Verification items for this drawing (mm, ordinates from the low corner). A direction names the side the tool comes from. Give positions to 0.01 mm unless a question says otherwise; leave off trailing zeros. Order: outer loops, then holes, each group sorted by start corner. A loop starts at its lowest first (then second) coordinate and runs counter-clockwise, first axis right, second up. Notation, with made-up numbers: M 36,68.5 L 71,68.5 A28 ccw 71,98.5 Z; hole C 84.5,-37.5 d9. An arc over 180 degrees is marked long. Answer as a JSON object with one key per item and string values.
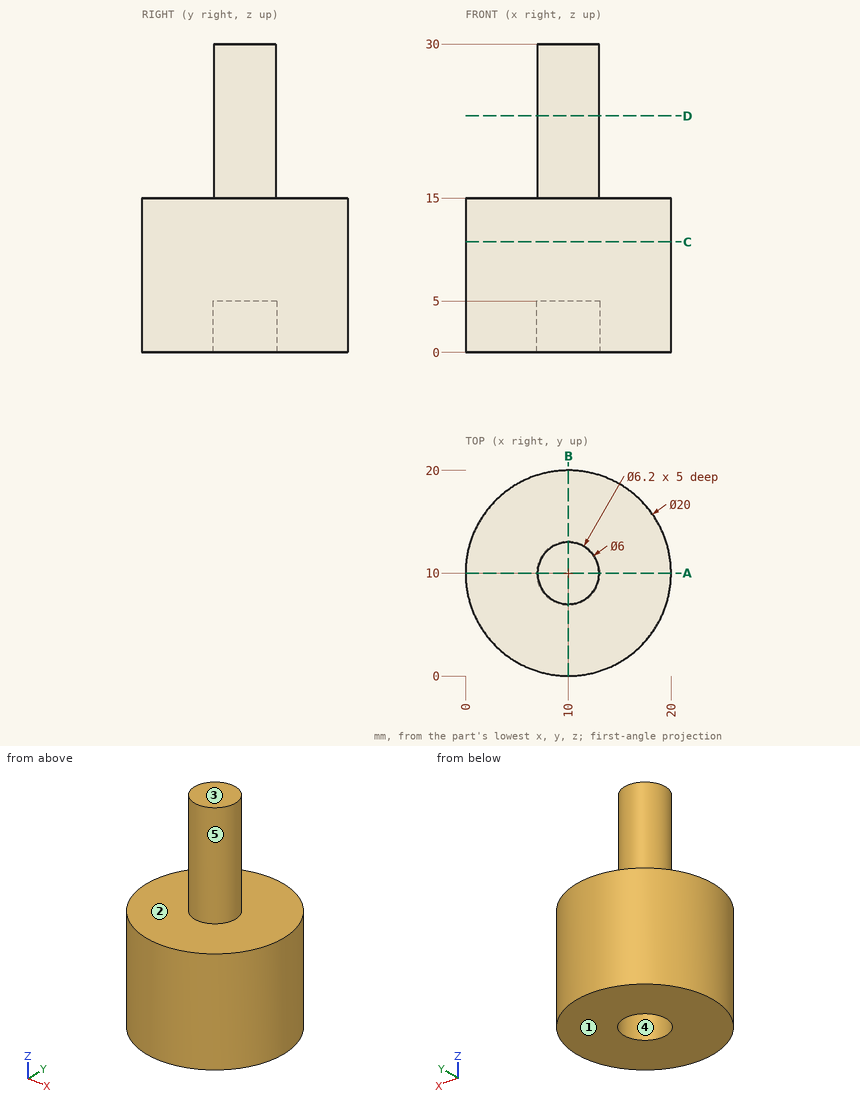
Q1. Material ranges on L1, parallel to Y at x = 10, z = 3.6; L2, parallel to Z at x = 3.25, y = 9.5; L3, parallel to X at y = 10.5, z = 1.75, recorded low to high.
Resolved:
{"L1": "y = 0 to 6.9, 13.1 to 20", "L2": "z = 0 to 15", "L3": "x = 0.01 to 6.94, 13.06 to 19.99"}
Q2. Tool access check on the marked faces 1 and 2. Record the directions out of +Z, -Z, +X, -X, +Y, -Y that give a thin tool (end or side, any length) a straight path to the whole face; none if there is none.
Resolved:
{"face 1": "-Z, +X, -X, +Y, -Y", "face 2": "+Z"}
Q3. Section check A-A on y = 10. Record the cut outline in (x, z).
Resolved:
{"outline": "M 0,0 L 6.9,0 L 6.9,5 L 13.1,5 L 13.1,0 L 20,0 L 20,15 L 13,15 L 13,30 L 7,30 L 7,15 L 0,15 Z"}
Q4. Release check for a two-part mould opening along X. For the marked faces 3, 4 and 5 record: +X half, -X half, draft (parallel to the pull), parting line (faces both ways), or undercut.
Resolved:
{"face 3": "draft", "face 4": "undercut", "face 5": "parting line"}
Q5. Gauge pin test, flat ends, axial feed: pin 1 Ø1 at (y, z) = (12, 5) entering from -X; pin 2 Ø3 at (x, y) = (8.5, 15.5) entering from +Z; pin 3 Ø8 at (x, z) = (16, 9) entering from +Y. Record the tip position at first contact, or that the pin passes through.
Resolved:
{"pin 1": "stops at x = 0.11", "pin 2": "stops at z = 15", "pin 3": "stops at y = 19.8"}
Q6. Section check C-C on z = 10.75. Record the cut outline in (x, y), then the cut area to 3 significant figures.
Resolved:
{"outline": "C 10,10 d20", "area": "314 mm²"}
Q7. Section check D-D on z = 23. Record the cut outline in (x, y), then the cut area to 3 significant figures.
Resolved:
{"outline": "C 10,10 d6", "area": "28.3 mm²"}
